Input: dimensioned drawing with shaded views. Units: mm. Origin: part minimum x, y, z. A direction names the side the tool comes from. Round coordinates to 2 decimals unless told otherwise and drop trailing zeros. Order: outer loops, then holes, each group sorted by start corner. A loop starts at its lowest first (then second) coordinate and runs counter-clockwise, first axis right, second up. Notation, with made-up numbers: M 9,28 L 38,28 A18 cw 38,55 Z; hole C 38,-18.75 d10. An arc over 180 degrees is marked long. Put each result on its own line as item: value. Start each with the question number.
1) Section D-D, the plane y = 43.5. Return loops of the section in (x, z) (3 decimals).
2) Access query for the marked faces 5, 6 and 7. Directions: +Z, -Z, +X, -X, +Y, -Y. A direction counts if a zero-diameter tool reaches every point of the face in a straight line with its end or side. Return the directions, or none.
3) Section B-B, the plane x = 33. Return loops of the section in (y, z).
4) First-contact query: P1, Ø17.5, axis at x = 98.5, y = 29, coming from the +Z side; P2, Ø9.5, axis at y = 33, z = 51.5, coming from the +X side; P3, Ø12, axis at x = 40.5, z = 44, coming from the -Y side; P4, Ø8, axis at x = 81.5, z = 52.5, coming from the +Y side. Flat tips, straight axial feed; report the tip coordinate or a pass-through.
5) Section A-A, the plane x = 62.5. Return loops of the section in (y, z), then the cut area to 3 significant figures.
6) Draft query along X for the marked faces 1, 2, 3 and 4. Return one class per face: pulls with the +X half, pulls with the -X half, needs draft (parallel to the pull), parting line crosses it, or undercut.
7) Material intervals for probe 1 along Z at (x, y) = (67.5, 29); probe 2 along Z at (x, y) = (67, 15); probe 3 along Y at (x, z) = (39, 18), sorted ascending. Write a range as [from, to].
8) Section C-C, the plane z = 24. Return loops of the section in (x, y), then the cut area to 3 significant figures.
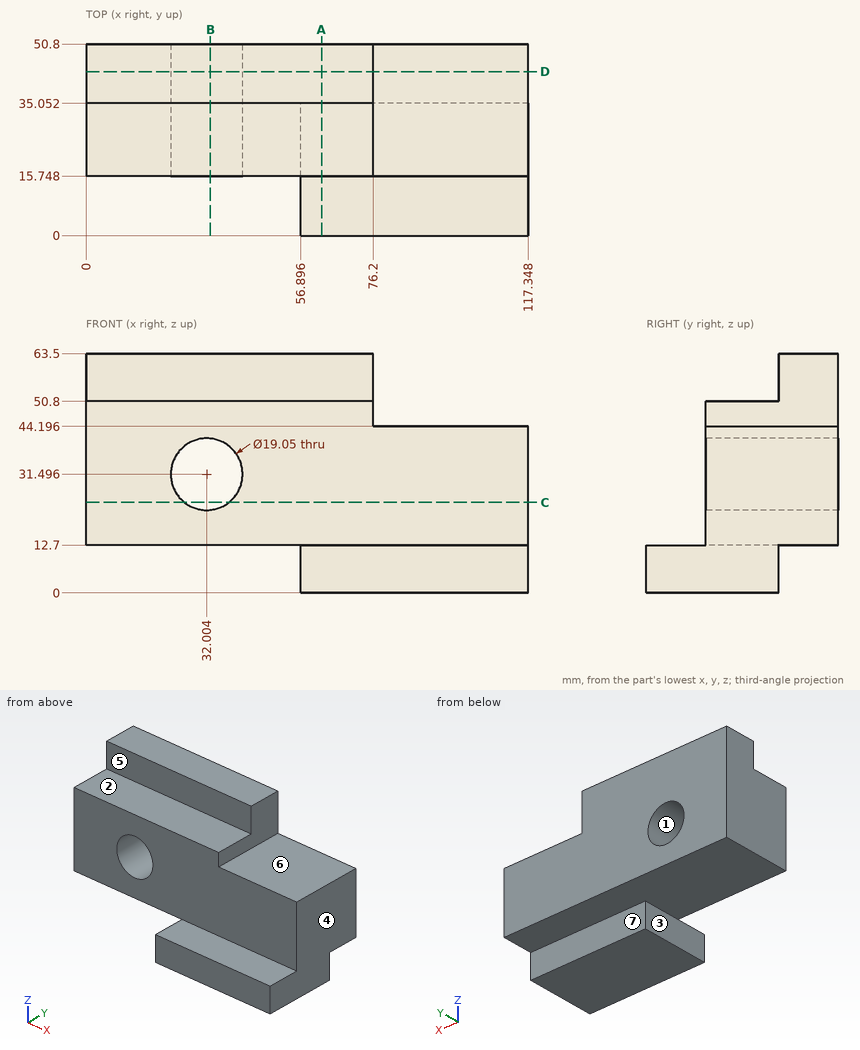
Result sheet:
1. outline: M 0,12.7 L 117.348,12.7 L 117.348,44.196 L 76.2,44.196 L 76.2,63.5 L 0,63.5 Z; hole C 32.004,31.496 d19.05
2. face 5: +Z, +X, -X, -Y
2. face 6: +Z, +X, +Y, -Y
2. face 7: -Z, +X, -X, +Y
3. outline: M 15.75,12.7 L 50.8,12.7 L 50.8,22.02 L 15.75,22.02 Z; M 15.75,40.97 L 50.8,40.97 L 50.8,63.5 L 35.05,63.5 L 35.05,50.8 L 15.75,50.8 Z
4. P1: stops at z = 44.2
4. P2: stops at x = 76.2
4. P3: stops at y = 15.75
4. P4: passes through
5. outline: M 0,0 L 35.05,0 L 35.05,12.7 L 50.8,12.7 L 50.8,63.5 L 35.05,63.5 L 35.05,50.8 L 15.75,50.8 L 15.75,12.7 L 0,12.7 Z
5. area: 1,980 mm2
6. face 1: undercut
6. face 2: needs draft
6. face 3: pulls with the -X half
6. face 4: pulls with the +X half
7. probe 1: z = [0, 50.8]
7. probe 2: z = [0, 12.7]
7. probe 3: y = [15.75, 50.8]
8. outline: M 0,15.75 L 26.13,15.75 L 26.13,50.8 L 0,50.8 Z; M 37.88,15.75 L 117.35,15.75 L 117.35,50.8 L 37.88,50.8 Z
8. area: 3,700 mm2
